Here's how the part is built. I have some questions about the finished solid (model axes, mm). Face numbers are marked on the shaded views. A direction names the side the tool comes from. Coordinates: 2 decimals unless noted, no trailing zeros. Write each loop counter-clockwise with the first axis right and the second up, starting at its lowest first coordinate (ties: lowest second). Pieces come first, ordered by that corner, then holes. Notation, with made-up numbers: M -20.75,79 L -2.75,79 A27 ccw -2.75,111 Z; hole C 9,-16.5 d2. An arc over 180 degrees is marked long. Use one line per item in the form item = value. Start each with the question number.
1. I want a section at C-C, the plane z = 1.5. Count the separate pieces of the cut face and the enclosed holes in it, plus the area to 3 significant figures.
2. Thinking about a two-plate mould opening in Y: for the marked faces 3, 4 and 5, which applies, released by +Y, released by -Y, zero draft, split by the parting line, or undercut?
3. I'm going to push flat-ended pins straight in: pin 1 Ø2.5 at (x, z) = (-2.5, 4.5) entering from -Y; pin 2 Ø3 at (x, z) = (-12.5, 3.5) entering from -Y; pin 3 Ø4 at (x, z) = (-30, 1.5) entering from -Y. Where does each tip first touch, or does it pass through?
4. Please list where these lines run through material, in increasing order: line 1 along Y through (x, z) = (-5.5, 2.25); line 2 along Y through (x, z) = (-15, 3.5); line 3 along Y through (x, z) = (-20.5, 5). Write a range as [from, to].
5. I want a section at B-B, the plane y = 76. List the corners of the cut face in (x, z) for me.
6. On a 3-axis mill with a long thin cutter (end or side, diameter ignored), from which of +Z, -Z, +X, -X, +Y, -Y can I reach the whole of each face in a straight line? I mean the marked faces 1 and 2. Say none if no direction works.
7. I want a section at A-A, the plane x = -5.5. List the corners of the cut face in (y, z) for me.
from build123d import *

# Parameters (mm, degrees)
SKETCH1_R           = 2.1
BOSS_EXTRUDE1_DEPTH = 8
CUT_EXTRUDE1_REACH  = 49.49
SKETCH2_R           = 1.65


with BuildPart() as part:
    # Sketch1 → Boss-Extrude1 (new body)
    with BuildSketch(Plane.XY):
        Polygon((-14.353967242, 72.5), (5, 72.5), (5, 80), (-19.131994198, 80), (-12.334685795, 76.830363037), align=None)
        with Locations((0, 76)):
            Circle(SKETCH1_R, mode=Mode.SUBTRACT)
        Polygon((-19.131994198, 72.5), (-14.353967242, 72.5), (-12.334685795, 76.830363037), (-19.131994198, 80), align=None)
        with BuildLine():
            Line((-30.628506806, 37.599137276), (-14.353967242, 72.5))
            Line((-14.353967242, 72.5), (-19.131994198, 72.5))
            Line((-19.131994198, 72.5), (-19.131994198, 80))
            Line((-19.131994198, 80), (-38.637128487, 38.171104532))
            ThreePointArc((-38.637128487, 38.171104532), (-35.992554118, 40.259685439), (-32.739034841, 39.381872183))
            ThreePointArc((-32.739034841, 39.381872183), (-31.696306875, 38.475663662), (-30.628506806, 37.599137276))
        make_face()
        with BuildLine():
            Line((-31.819822815, 35.044351851), (-30.628506806, 37.599137276))
            ThreePointArc((-30.628506806, 37.599137276), (-31.696306875, 38.475663662), (-32.739034841, 39.381872183))
            ThreePointArc((-32.739034841, 39.381872183), (-35.992554118, 40.259685439), (-38.637128487, 38.171104532))
            ThreePointArc((-38.637128487, 38.171104532), (-38.911873793, 35.832206175), (-37.737913805, 33.790699757))
            ThreePointArc((-37.737913805, 33.790699757), (-37.315296786, 33.416625413), (-36.888971991, 33.046782299))
            Line((-36.888971991, 33.046782299), (-33.490317789, 31.461963818))
            Line((-33.490317789, 31.461963818), (-32.97126033, 32.575086132))
            ThreePointArc((-32.97126033, 32.575086132), (-32.850330683, 34.021790637), (-31.819822815, 35.044351851))
        make_face()
        with Locations((-35.238474323, 36.58628597)):
            Circle(SKETCH1_R, mode=Mode.SUBTRACT)
        with BuildLine():
            ThreePointArc((0, 26.880434783), (-16.224950018, 29.637486219), (-30.628506806, 37.599137276))
            Line((-30.628506806, 37.599137276), (-31.819822815, 35.044351851))
            ThreePointArc((-31.819822815, 35.044351851), (-29.811908313, 34.901033754), (-28.847084331, 33.134292287))
            ThreePointArc((-28.847084331, 33.134292287), (-30.664922673, 31.053334623), (-32.97126033, 32.575086132))
            Line((-32.97126033, 32.575086132), (-33.490317789, 31.461963818))
            Line((-33.490317789, 31.461963818), (-36.888971991, 33.046782299))
            ThreePointArc((-36.888971991, 33.046782299), (-19.669553306, 22.906838122), (0, 19.380434783))
            ThreePointArc((0, 19.380434783), (3.75, 23.130434783), (0, 26.880434783))
        make_face()
        with Locations((-26.319869018, 30.147460036)):
            Circle(SKETCH1_R, mode=Mode.SUBTRACT)
        with Locations((-21.407041065, 27.658201118)):
            Circle(SKETCH1_R, mode=Mode.SUBTRACT)
        with Locations((-16.261912507, 25.693527972)):
            Circle(SKETCH1_R, mode=Mode.SUBTRACT)
        with Locations((-10.940316211, 24.274760441)):
            Circle(SKETCH1_R, mode=Mode.SUBTRACT)
        with Locations((-5.5, 23.417294418)):
            Circle(SKETCH1_R, mode=Mode.SUBTRACT)
        with Locations((0, 23.130434783)):
            Circle(SKETCH1_R, mode=Mode.SUBTRACT)
    extrude(amount=BOSS_EXTRUDE1_DEPTH)

    # Sketch2 → Cut-Extrude1 (cut, up to next)
    with BuildSketch(Plane(origin=(-46.356679233, 21.616474533, 0), x_dir=(0, 0, 1), z_dir=(-0.906307787, 0.422618262, 0)), mode=Mode.PRIVATE) as cut_extrude1_sk1:
        with Locations((4, 55.04255297)):
            Circle(SKETCH2_R)
    cut_extrude1_tool1 = extrude(cut_extrude1_sk1.sketch, amount=-CUT_EXTRUDE1_REACH, mode=Mode.PRIVATE) & part.part
    add(cut_extrude1_tool1.solids().sort_by_distance((-23.094691, 71.501969, 4))[0], mode=Mode.SUBTRACT)
    # Sketch2 → Cut-Extrude1 (cut, up to next)
    with BuildSketch(Plane(origin=(-46.356679233, 21.616474533, 0), x_dir=(0, 0, 1), z_dir=(-0.906307787, 0.422618262, 0)), mode=Mode.PRIVATE) as cut_extrude1_sk2:
        with Locations((4, 27.64255297)):
            Circle(SKETCH2_R)
    cut_extrude1_tool2 = extrude(cut_extrude1_sk2.sketch, amount=-CUT_EXTRUDE1_REACH, mode=Mode.PRIVATE) & part.part
    add(cut_extrude1_tool2.solids().sort_by_distance((-34.674432, 46.669136, 4))[0], mode=Mode.SUBTRACT)


solid = part.part
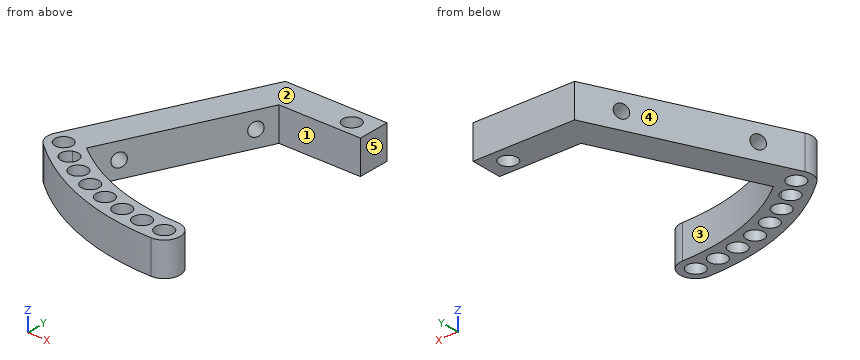
Answer list:
q1.separate_pieces = 1
q1.enclosed_holes = 9
q1.area = 676 mm²
q2.face_3 = undercut
q2.face_4 = released by +Y
q2.face_5 = zero draft
q3.pin_1 = 19.39
q3.pin_2 = 20.46
q3.pin_3 = 26.79
q4.line_1 = [19.65, 21.32], [25.52, 27.19], [72.5, 80]
q4.line_2 = [21.4, 24.01], [27.37, 29.23], [71.11, 80]
q4.line_3 = [23.22, 25.76], [29.55, 31.36], [59.32, 68.84], [71.74, 77.07]
q5.outline = M -21,0 L -2.1,0 L -2.1,8 L -21,8 Z; M 2.1,0 L 5,0 L 5,8 L 2.1,8 Z
q6.face_1 = +Z, -Z, +X
q6.face_2 = +Z, +X, -X, +Y, -Y
q7.outline = M 19.65,0 L 21.32,0 L 21.32,8 L 19.65,8 Z; M 25.52,0 L 27.19,0 L 27.19,8 L 25.52,8 Z; M 72.5,0 L 80,0 L 80,8 L 72.5,8 Z
